For this review, use the dimensioned drawing (mm, ordinates from the lowest corner) and the shaded views. A direction names the side the tool comes from. Coordinates: 2 decimals unless noted, no trailing zeros. Order: outer loops, then holes, each group sorted by start corner. A loop starts at its lowest first (then second) coordinate and runs counter-clockwise, first axis right, second up. Notation, with made-up numbers: M 41.5,83.25 L 59.5,83.25 A21 ccw 59.5,108.25 Z; hole C 57,75 d1. An arc over 180 degrees is marked long. Use CSV: the item, a comma, the result in double quotes.
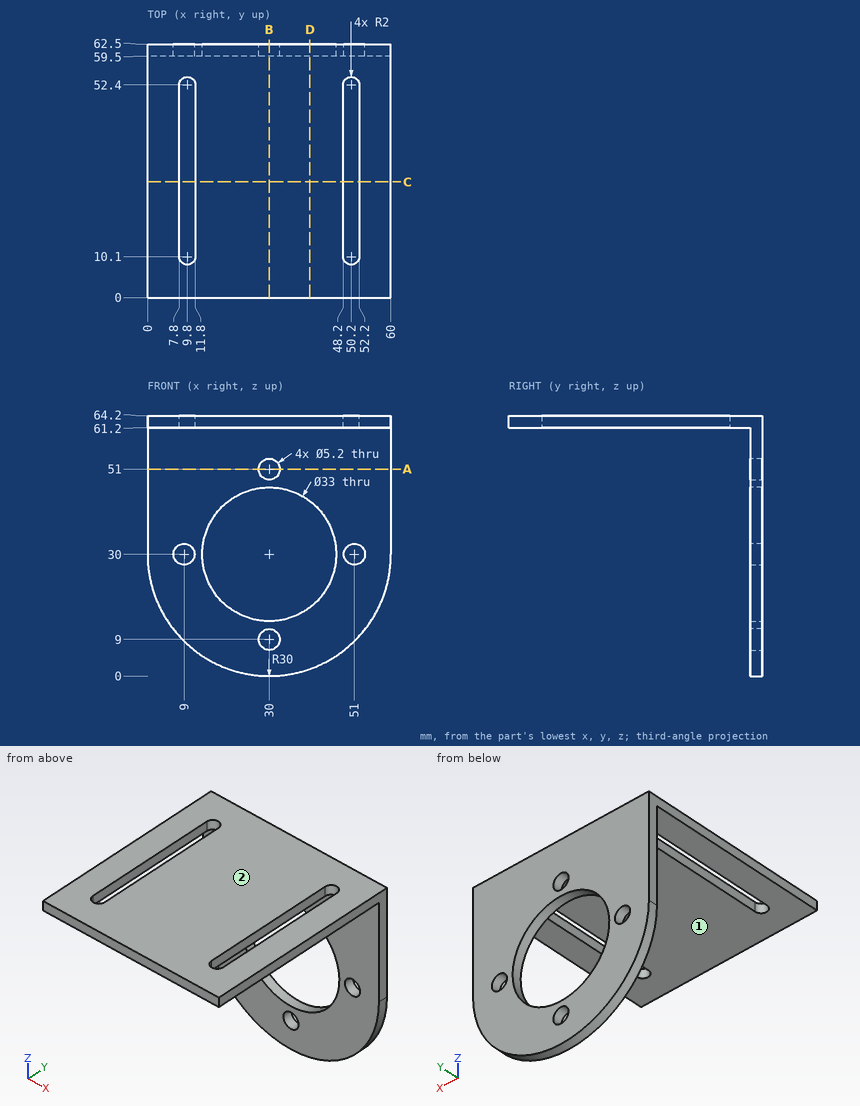
Item 1: Add section A-A on z = 51. State the section outline as (x, y) points, and give its area (3 significant figures).
Solutions:
outline,"M 0,59.5 L 27.4,59.5 L 27.4,62.5 L 0,62.5 Z; M 32.6,59.5 L 60,59.5 L 60,62.5 L 32.6,62.5 Z"
area,"164 mm^2"
Item 2: For the marked faces 1 and 2, list the 3-axis set-ups (+Z, -Z, +X, -X, +Y, -Y) from which the entire face can be reached by the end or side of a thin tool; tool diameter is ignored.
Solutions:
face 1,"-Z, +X, -X, -Y"
face 2,"+Z, +X, -X, +Y, -Y"
Item 3: Clearance check with flat-ended pins moving along their axes: pin 1 Ø7 at (x, z) = (30, 9) entering from -Y; pin 2 Ø1 at (x, y) = (19, 35) entering from -Z. State where each tip first meets the part, or that it passes through.
Solutions:
pin 1,"y = 59.5"
pin 2,"z = 61.2"
Item 4: Add section B-B on x = 30. State the section outline as (y, z) points.
Solutions:
outline,"M 0,61.2 L 59.5,61.2 L 59.5,53.6 L 62.5,53.6 L 62.5,64.2 L 0,64.2 Z; M 59.5,0 L 62.5,0 L 62.5,6.4 L 59.5,6.4 Z; M 59.5,11.6 L 62.5,11.6 L 62.5,13.5 L 59.5,13.5 Z; M 59.5,46.5 L 62.5,46.5 L 62.5,48.4 L 59.5,48.4 Z"
Item 5: To check wall thickness, follow line 1 along X through (y, z) = (60.7, 30); line 2 along X through (y, z) = (61.1, 51); line 3 along Z through (x, y) = (25.5, 46). State the ranges of each line that lie inside material, in increasing order. Write a range as [from, to].
Solutions:
line 1,"[0, 6.4], [11.6, 13.5], [46.5, 48.4], [53.6, 60]"
line 2,"[0, 27.4], [32.6, 60]"
line 3,"[61.2, 64.2]"
Item 6: Add section C-C on y = 28.5. State the section outline as (x, z) points.
Solutions:
outline,"M 0,61.2 L 7.8,61.2 L 7.8,64.2 L 0,64.2 Z; M 11.8,61.2 L 48.2,61.2 L 48.2,64.2 L 11.8,64.2 Z; M 52.2,61.2 L 60,61.2 L 60,64.2 L 52.2,64.2 Z"
Item 7: Add section D-D on x = 40. State the section outline as (y, z) points, and give its area (3 significant figures).
Solutions:
outline,"M 0,61.2 L 59.5,61.2 L 59.5,43.12 L 62.5,43.12 L 62.5,64.2 L 0,64.2 Z; M 59.5,1.72 L 62.5,1.72 L 62.5,16.88 L 59.5,16.88 Z"
area,"287 mm^2"
